Input: part model. Units: mm. Frame: model coordinates. A direction names the side the tool comes from. Give positions to 0.01 mm unless a question says otherwise; leave off trailing zeros. Loops run counter-clockwise (first coordinate to the right, second up) from the corner with the lowest first, then second, coordinate; pieces in that order, holes last. Notation, with made-up numbers: (30.5, 75.5) - (80.5, 75.5) arc R10 ccw to (80.5, 94.5) - close; hole circle Ø6 at (-6.75, 8). An arc over 180 degrees is marked (long way). Answer as a JSON object with one key per item and string values. Group by question number.
(1) Section query B-B (x = 100). Return loops of the section in (y, z), plus the area to 3 significant figures.
(2) Access query for faces 1 (the flat face through (100, 0, -140)), 2 (the flat face through (101, 101.6, -102)), 3 (the flat face through (103, 50, -25.4)), 4 (the flat face through (103, 25, -127)), 5 (the flat face through (100, 13, 0)). Directions: +Z, -Z, +X, -X, +Y, -Y. A direction counts if a zero-diameter tool reaches every point of the face in a straight line with its end or side. Return the directions, or none.
(3) Section query D-D (y = 139). Return loops of the section in (x, z), plus the area to 3 significant figures.
(4) Mould query, pull axis X, two halves, no side actions, for faces 6 (the flat face through (103, 25.4, -13)), 7 (the flat face through (0, 75, -92)), 8 (the flat face through (127, 127, -101)). Classes: +X half, -X half, draft (parallel to the pull), parting line (faces both ways), or undercut.
(5) Pin query (flat end, axial travel): P1, Ø15, axis at x = 94.5, y = 115.5, coming from the +Z side; P2, Ø3, axis at x = 131.5, z = -121, coming from the -Y side; P3, Ø20.5, axis at x = 122, z = -19, coming from the +Y side. Return the tip coordinate at first contact, or that it passes through.
(6) Section query C-C (z = -92). Return loops of the section in (x, y), plus the area to 3 significant figures.
(7) Section query A-A (y = 36.5). Return loops of the section in (x, z), plus the area to 3 significant figures.
(8) Material intervals for L1, parallel to Z at x = 82.5, y = 29; L2, parallel to X at y = 102, z = -108.5; L3, parallel to Z at x = 155.5, y = 8, sorted ascending.
```python
from build123d import *

# Parameters (mm, degrees)
SKETCH1_W           = 203.2
SKETCH1_H           = 152.4
BOSS_EXTRUDE1_DEPTH = 152.4
SKETCH2_W           = 50.8
SKETCH2_H           = 50.8
CUT_EXTRUDE1_DEPTH  = 204.2
SKETCH3_W           = 50.8
SKETCH3_H           = 50.8
CUT_EXTRUDE2_DEPTH  = 50.8


with BuildPart() as part:
    # Sketch1 → Boss-Extrude1 (new body)
    with BuildSketch(Plane.XY):
        with Locations((101.6, 76.2)):
            Rectangle(SKETCH1_W, SKETCH1_H)
    extrude(amount=-BOSS_EXTRUDE1_DEPTH)

    # Sketch2 → Cut-Extrude1 (cut, through all)
    with BuildSketch(Plane(origin=(203.2, 0, 0), x_dir=(0, 0, -1), z_dir=(1, 0, 0))):
        Polygon((0, 25.4), (25.4, 25.4), (25.4, 76.2), (76.2, 76.2), (76.2, 152.4), (0, 152.4), align=None)
        with Locations((101.6, 25.4)):
            Rectangle(SKETCH2_W, SKETCH2_H)
    extrude(amount=-CUT_EXTRUDE1_DEPTH, mode=Mode.SUBTRACT)

    # Sketch3 → Cut-Extrude2 (cut)
    with BuildSketch(Plane(origin=(0, 152.4, 0), x_dir=(1, 0, 0), z_dir=(0, 1, 0))):
        with Locations((101.6, 101.6)):
            Rectangle(SKETCH3_W, SKETCH3_H)
    extrude(amount=-CUT_EXTRUDE2_DEPTH, mode=Mode.SUBTRACT)


solid = part.part
```
Recorded:
{
 "1": {"outline": "(0, -152.4) - (152.4, -152.4) - (152.4, -127) - (101.6, -127) - (101.6, -76.2) - (76.2, -76.2) - (76.2, -25.4) - (25.4, -25.4) - (25.4, 0) - (0, 0) - (0, -76.2) - (50.8, -76.2) - (50.8, -127) - (0, -127) - close", "area": "11,000 mm^2"},
 "2": {"face 1": "+Z, -Z, +X, -X, -Y", "face 2": "+Z, +Y", "face 3": "+Z, +X, -X, +Y", "face 4": "+X, -X, -Y", "face 5": "+Z, +X, -X, +Y, -Y"},
 "3": {"outline": "(0, -152.4) - (203.2, -152.4) - (203.2, -76.2) - (127, -76.2) - (127, -127) - (76.2, -127) - (76.2, -76.2) - (0, -76.2) - close", "area": "12,900 mm^2"},
 "4": {"face 6": "draft", "face 7": "-X half", "face 8": "undercut"},
 "5": {"P1": "stops at z = -127", "P2": "stops at y = 50.8", "P3": "stops at y = 76.2"},
 "6": {"outline": "(0, 50.8) - (203.2, 50.8) - (203.2, 152.4) - (127, 152.4) - (127, 101.6) - (76.2, 101.6) - (76.2, 152.4) - (0, 152.4) - close", "area": "18,100 mm^2"},
 "7": {"outline": "(0, -152.4) - (203.2, -152.4) - (203.2, -127) - (0, -127) - close; (0, -76.2) - (203.2, -76.2) - (203.2, -25.4) - (0, -25.4) - close", "area": "15,500 mm^2"},
 "8": {"L1": "z = -152.4 to -127, -76.2 to -25.4", "L2": "x = 0 to 76.2, 127 to 203.2", "L3": "z = -152.4 to -127, -76.2 to 0"}
}
